The listing builds one solid part. Answer for the finished solid, in the listing's coordinates (mm). A direction names the side the tool comes from. Round coordinates to 2 decimals unless told otherwise and drop trailing zeros. Order: outer loops, then holes, each group sorted by start corner. A loop starts at its lowest first (then second) coordinate and runs counter-clockwise, first axis right, second up. Notation, with made-up numbers: (10.5, -34) - (67.5, -34) arc R15 cw to (67.5, -15) - close; hole circle Ø6 at (14.25, 47). An arc over 180 degrees is marked (long way). Use CSV: the item, a comma, the result in double quotes. Start each with the question number.
Item 1: Flat-ended cylindrical pins translate along their axes: P1, Ø1, axis at x = -2.5, y = -1.5, coming from the +Z side; P2, Ø8, axis at x = 17, y = -7, coming from the -Z side. Find the tip coordinate at first contact, or state that the pin passes through.
Item 2: Find section B-B, the plane x = 7. Give the vertices of the cut face in (y, z), plus the area to 3 significant figures.
Item 3: Determine the mould class of faces 3 (the flat face through (-1, -35, 14)), 4 (the cylindrical face through (54.1, -34.14, 13.56)), 5 (the cylindrical face through (-48.665, -28.759, 14.825)) for opening direction X: +X half, -X half, draft (parallel to the pull), parting line (faces both ways), or undercut.
Item 4: Find section D-D, the plane z = 9. Give the vertices of the cut face in (x, y).
Item 5: Find section C-C, the plane z = 3.75. Give the vertices of the cut face in (x, y), plus the area to 3 significant figures.
Item 6: For faces 1 (the flat face through (-51, -31, 2.5)), 2 (the cylindrical face through (-54.14, -34.1, 13.56)), determine the directions among +Z, -Z, +X, -X, +Y, -Y from which every point of the face is accessible in a straight line to the end or side of a thin tool.
Item 7: Find section A-A, the plane y = -7. Give the vertices of the cut face in (x, z), plus the area to 3 significant figures.
Item 8: Straight lines are drawn through the part: line 1 along Y through (x, z) = (-17, 18); line 2 along X through (y, z) = (18, 18); line 3 along Z through (x, y) = (16, -15.5). For each, find the intervals that lie inside material, in ascending order. Write a range as [from, to].
```python
from build123d import *

# Parameters (mm, degrees)
F0_W     = 106
F0_H     = 66
F1_DEPTH = 2.5
F2_DEPTH = 27.5
F3_R     = 3.65
F3_R_2   = 1
F4_DEPTH = 25
F7_DEPTH = 2


with BuildPart() as f1:
    # F0 (on Top) → F1 (new body)
    with BuildSketch(Plane.XY):
        with BuildLine():
            ThreePointArc((55, 32), (54.12132, 34.12132), (52, 35))
            Line((52, 35), (-52, 35))
            ThreePointArc((-52, 35), (-54.12132, 34.12132), (-55, 32))
            Line((-55, 32), (-55, -32))
            ThreePointArc((-55, -32), (-54.12132, -34.12132), (-52, -35))
            Line((-52, -35), (52, -35))
            ThreePointArc((52, -35), (54.12132, -34.12132), (55, -32))
            Line((55, -32), (55, 32))
        make_face()
        Rectangle(F0_W, F0_H, mode=Mode.SUBTRACT)
        Rectangle(F0_W, F0_H)
    extrude(amount=F1_DEPTH)

    # F0 (on Top) → F2 (join)
    with BuildSketch(Plane.XY):
        with BuildLine():
            ThreePointArc((55, 32), (54.12132, 34.12132), (52, 35))
            Line((52, 35), (-52, 35))
            ThreePointArc((-52, 35), (-54.12132, 34.12132), (-55, 32))
            Line((-55, 32), (-55, -32))
            ThreePointArc((-55, -32), (-54.12132, -34.12132), (-52, -35))
            Line((-52, -35), (52, -35))
            ThreePointArc((52, -35), (54.12132, -34.12132), (55, -32))
            Line((55, -32), (55, 32))
        make_face()
        Rectangle(F0_W, F0_H, mode=Mode.SUBTRACT)
    extrude(amount=F2_DEPTH)

    # F3 (on face) → F4 (join)
    with BuildSketch(Plane.XY.offset(2.5)):
        with Locations((-51.286835, 31.298466)):
            Circle(F3_R)
        with Locations((-51.286835, 31.298466)):
            Circle(F3_R_2, mode=Mode.SUBTRACT)
        with Locations((-51.286835, -31.298466)):
            Circle(F3_R)
        with Locations((-51.286835, -31.298466)):
            Circle(F3_R_2, mode=Mode.SUBTRACT)
        with Locations((51.286835, -31.298466)):
            Circle(F3_R)
        with Locations((51.286835, -31.298466)):
            Circle(F3_R_2, mode=Mode.SUBTRACT)
        with Locations((51.286835, 31.298466)):
            Circle(F3_R)
        with Locations((51.286835, 31.298466)):
            Circle(F3_R_2, mode=Mode.SUBTRACT)
    extrude(amount=F4_DEPTH)

    # F6 (on offset) → F7 (cut, through all)
    with BuildSketch(Plane.XZ.offset(35)):
        with BuildLine():
            Line((-2.5, 2.5), (2.5, 2.499828))
            ThreePointArc((2.5, 2.499828), (8.6e-05, 5), (-2.5, 2.5))
        make_face()
    extrude(amount=-F7_DEPTH, mode=Mode.SUBTRACT)


solid = f1.part
```
Worked out:
1,P1,"stops at z = 2.5"
1,P2,"stops at z = 0"
2,outline,"(-35, 0) - (35, 0) - (35, 27.5) - (33, 27.5) - (33, 2.5) - (-33, 2.5) - (-33, 27.5) - (-35, 27.5) - close"
2,area,"275 mm²"
3,face 3,"draft"
3,face 4,"+X half"
3,face 5,"undercut"
4,outline,"(-55, -32) arc R3 ccw to (-52, -35) - (52, -35) arc R3 ccw to (55, -32) - (55, 32) arc R3 ccw to (52, 35) - (-52, 35) arc R3 ccw to (-55, 32) - close; hole (-53, -28.08) arc R3.65 cw to (-48.06, -33) - (48.06, -33) arc R3.65 cw to (53, -28.08) - (53, 28.08) arc R3.65 cw to (48.06, 33) - (-48.06, 33) arc R3.65 cw to (-53, 28.08) - close; hole circle Ø2 at (-51.29, -31.3); hole circle Ø2 at (-51.29, 31.3); hole circle Ø2 at (51.29, -31.3); hole circle Ø2 at (51.29, 31.3)"
5,outline,"(-55, -32) arc R3 ccw to (-52, -35) - (-2.17, -35) - (-2.17, -33) - (-48.06, -33) arc R3.65 ccw to (-53, -28.08) - (-53, 28.08) arc R3.65 ccw to (-48.06, 33) - (48.06, 33) arc R3.65 ccw to (53, 28.08) - (53, -28.08) arc R3.65 ccw to (48.06, -33) - (2.17, -33) - (2.17, -35) - (52, -35) arc R3 ccw to (55, -32) - (55, 32) arc R3 ccw to (52, 35) - (-52, 35) arc R3 ccw to (-55, 32) - close; hole circle Ø2 at (-51.29, -31.3); hole circle Ø2 at (-51.29, 31.3); hole circle Ø2 at (51.29, -31.3); hole circle Ø2 at (51.29, 31.3)"
5,area,"777 mm²"
6,face 1,"+Z"
6,face 2,"+Z, -Z, -X, -Y"
7,outline,"(-55, 0) - (55, 0) - (55, 27.5) - (53, 27.5) - (53, 2.5) - (-53, 2.5) - (-53, 27.5) - (-55, 27.5) - close"
7,area,"375 mm²"
8,line 1,"y = [-35, -33], [33, 35]"
8,line 2,"x = [-55, -53], [53, 55]"
8,line 3,"z = [0, 2.5]"
